Build history of the part. All positions in model axes, mm. A direction names the side the tool comes from. Coordinates: 2 decimals unless noted, no trailing zeros. Write each loop counter-clockwise with the first axis right and the second up, starting at its lowest first coordinate (ties: lowest second). Pieces come first, ordered by that corner, then holes.
```python
from build123d import *

# Parameters (mm, degrees)
F0_R     = 63.5
F1_DEPTH = 508
F3_R     = 127
F4_DEPTH = 127


with BuildPart() as f1:
    # F0 (on Top) → F1 (new body)
    with BuildSketch(Plane.XY):
        Circle(F0_R)
    extrude(amount=F1_DEPTH)

    # F3 (on offset) → F4 (join)
    with BuildSketch(Plane(origin=(0, 0, 127), x_dir=(1, 0, 0), z_dir=(0, 0, -1))):
        Circle(F3_R)
    extrude(amount=-F4_DEPTH)


solid = f1.part
```
1. 3-axis set-ups, long thin cutter, end or side, ignore diameter. For faces 1 (the face through (26.4, -58.2, 254)), 2 (the face through (26.4, -58.2, 127)), 3 (the face through (-27.53, 123.98, 189.61)): which of +Z, -Z, +X, -X, +Y, -Y reach the whole face in a straight line?
Computed values:
face 1: +Z
face 2: -Z
face 3: +Z, -Z
2. Probe line 1 along Z through (x, y) = (70, 99); line 2 along X through (y, z) = (9.5, 327); line 3 along Y through (x, z) = (-56, 419). List the from-to ranges inside material, lowest first.
Computed values:
line 1: z = 127 to 254
line 2: x = -62.79 to 62.79
line 3: y = -29.94 to 29.94
3. Flat gauge pins, fed straight in: pin 1 (5 mm diameter, centred on x = 34.5, y = 66, fed in from +Z); pin 2 (6 mm diameter, centred on x = 34, z = 341, fed in from +Y); pin 3 (10 mm diameter, centred on x = -46, z = 255, fed in from -Y). Where does each tip first touch, or does it go through?
Computed values:
pin 1: stops at z = 254
pin 2: stops at y = 55.42
pin 3: stops at y = -120.17
4. Saw through at D-D on x = -110. List the corners of the cut face in (y, z), plus the area to 3 significant figures.
Computed values:
outline: (-63.47, 127) - (63.47, 127) - (63.47, 254) - (-63.47, 254) - close
area: 16,100 mm2
5. Saw through at C-C on z = 431.5. List the corners of the cut face in (x, y), plus the area to 3 significant figures.
Computed values:
outline: circle Ø127 at (0, 0)
area: 12,700 mm2
6. Saw through at A-A on x = 0. List the corners of the cut face in (y, z), plus the area to 3 significant figures.
Computed values:
outline: (-127, 127) - (-63.5, 127) - (-63.5, 0) - (63.5, 0) - (63.5, 127) - (127, 127) - (127, 254) - (63.5, 254) - (63.5, 508) - (-63.5, 508) - (-63.5, 254) - (-127, 254) - close
area: 80,600 mm2
